```python
from build123d import *

# Parameters (mm, degrees)
BOX_W           = 45
BOX_H           = 29
BOX_DEPTH       = 7.2
SKETCH_R        = 1.68
POCKET_DEPTH    = 29.001
SKETCH001_R     = 9.3
SKETCH001_W     = 10
SKETCH001_H     = 21
POCKET001_DEPTH = 8
FILLET_R        = 2
FILLET001_R     = 12.4


with BuildPart() as part:
    # Box → Box (new body)
    with BuildSketch(Plane.XY):
        with Locations((22.5, 14.5)):
            Rectangle(BOX_W, BOX_H)
    extrude(amount=BOX_DEPTH)

    # Sketch → Pocket (cut, through all)
    with BuildSketch(Plane.XZ):
        with Locations((6, 3.6)):
            Circle(SKETCH_R)
        with Locations((39, 3.6)):
            Circle(SKETCH_R)
    extrude(amount=-POCKET_DEPTH, mode=Mode.SUBTRACT)

    # Sketch001 → Pocket001 (cut)
    with BuildSketch(Plane.XY.offset(7.2)):
        with Locations((22.5, 15)):
            Circle(SKETCH001_R)
        with Locations((5, 18.5)):
            Rectangle(SKETCH001_W, SKETCH001_H)
        with Locations((40, 18.5)):
            Rectangle(SKETCH001_W, SKETCH001_H)
    extrude(amount=-POCKET001_DEPTH, mode=Mode.SUBTRACT)

    # Fillet
    fillet_edges = [part.edges().sort_by_distance(p)[0] for p in [
        (45, 8, 3.6),
        (35, 8, 3.6),
        (10, 8, 3.6),
        (0, 8, 3.6),
    ]]
    fillet(fillet_edges, radius=FILLET_R)

    # Fillet001
    fillet001_edges = [part.edges().sort_by_distance(p)[0] for p in [
        (10, 29, 3.6),
        (35, 29, 3.6),
    ]]
    fillet(fillet001_edges, radius=FILLET001_R)


solid = part.part
```
Model file for the job. Use its own axes, mm. A direction names the side the tool comes from. Coordinates: 2 decimals unless noted, no trailing zeros. Order: outer loops, then holes, each group sorted by start corner. A loop starts at its lowest first (then second) coordinate and runs counter-clockwise, first axis right, second up. Notation, with made-up numbers: (47, -27) -> (58, -27) arc R15 cw to (58, -15) -> close; hole circle Ø5 at (-15.75, 52). An arc over 180 degrees is marked (long way). Answer as a JSON object with one key per item and string values. Group by question number.
1) Cut at B-B, the plane x = 39. Write the cut outline in (y, z), then the cut area to 3 significant figures.
2) Pull direction Z, two halves, no side cores. Call faces 4 (the face through (22, 5, 7.2)), 5 (the face through (7.602, 3.944, 4.105)), 6 (the face through (9.4, 8.57, 3.55)): +Z half, -Z half, draft (parallel to the pull), parting line (faces both ways), or undercut.
3) Cut at A-A, the plane z = 3.6. Write the cut outline in (x, y).
4) Which spindle directions (+Z, -Z, +X, -X, +Y, -Y) get a long thin tool onto all of the face, cutting with end or side? Do faces 1 (the face through (4, 8, 4)), 2 (the face through (41, 8, 4)), 3 (the face through (45, 3, 4)). Say none if no direction does.
5) Cut at C-C, the plane y = 15. Write the cut outline in (x, z).
6) Drill centre lines: L1, parallel to Z at x = 6, y = 4.5; L2, parallel to X at y = 2.5, z = 4; L3, parallel to Y at x = 22.5, z = 4.25. Where is each one in solid material? Low to high.
7) Flat gauge pins, fed straight in: pin 1 (1.5 mm diameter, centred on y = 16.5, z = 1.5, fed in from -X); pin 2 (2 mm diameter, centred on x = 11, z = 2.5, fed in from -Y); pin 3 (1.8 mm diameter, centred on x = 40, z = 3, fed in from +Y); pin 4 (3.5 mm diameter, centred on y = 13.5, z = 4.5, fed in from +X). Where does each tip first touch, or does it go through?
8) Cut at D-D, the plane z = 1. Write the cut outline in (x, y), then the cut area to 3 significant figures.
Check values:
{
 "1": {"outline": "(0, 0) -> (8, 0) -> (8, 1.92) -> (0, 1.92) -> close; (0, 5.28) -> (8, 5.28) -> (8, 7.2) -> (0, 7.2) -> close", "area": "30.7 mm²"},
 "2": {"face 4": "+Z half", "face 5": "undercut", "face 6": "draft"},
 "3": {"outline": "(0, 0) -> (4.32, 0) -> (4.32, 8) -> (2, 8) arc R2 ccw to (0, 6) -> close; (7.68, 0) -> (37.32, 0) -> (37.32, 8) -> (37, 8) arc R2 cw to (35, 10) -> (35, 16.6) arc R12.4 ccw to (22.6, 29) -> (22.4, 29) arc R12.4 ccw to (10, 16.6) -> (10, 10) arc R2 cw to (8, 8) -> (7.68, 8) -> close; (40.68, 0) -> (45, 0) -> (45, 6) arc R2 ccw to (43, 8) -> (40.68, 8) -> close; hole circle Ø18.6 at (22.5, 15)"},
 "4": {"face 1": "+Z, -Z, -X, +Y", "face 2": "+Z, -Z, +X, +Y", "face 3": "+Z, -Z, +X, +Y, -Y"},
 "5": {"outline": "(10, 0) -> (13.2, 0) -> (13.2, 7.2) -> (10, 7.2) -> close; (31.8, 0) -> (35, 0) -> (35, 7.2) -> (31.8, 7.2) -> close"},
 "6": {"L1": "z = 0 to 1.92, 5.28 to 7.2", "L2": "x = 0 to 4.37, 7.63 to 37.37, 40.63 to 45", "L3": "y = 0 to 5.7, 24.3 to 29"},
 "7": {"pin 1": "stops at x = 10", "pin 2": "stops at y = 0", "pin 3": "stops at y = 8", "pin 4": "stops at x = 35"},
 "8": {"outline": "(0, 0) -> (45, 0) -> (45, 6) arc R2 ccw to (43, 8) -> (37, 8) arc R2 cw to (35, 10) -> (35, 16.6) arc R12.4 ccw to (22.6, 29) -> (22.4, 29) arc R12.4 ccw to (10, 16.6) -> (10, 10) arc R2 cw to (8, 8) -> (2, 8) arc R2 ccw to (0, 6) -> close; hole circle Ø18.6 at (22.5, 15)", "area": "547 mm²"}
}
